The listing builds one solid part. Answer for the finished solid, in the listing's coordinates (mm). A direction names the side the tool comes from. Round coordinates to 2 decimals unless told otherwise and drop trailing zeros. Write each loop counter-clockwise with the first axis right and the second up, starting at its lowest first coordinate (ties: lowest second). Pieces come first, ordered by that corner, then holes.
(1) For faces 4 (the face through (5.07, 345.49, -4.28)), 5 (the face through (25, 312, -25)), 6 (the face through (18, 121, -10)), determine the directions among +Z, -Z, +X, -X, +Y, -Y from which every point of the face is accessible in a straight line to the end or side of a thin tool.
(2) A cutting plane is placed at D-D, the plane x = 4.5. Give the vertices of the cut face in (y, z).
(3) A cutting plane is placed at C-C, the plane y = 325. Give the vertices of the cut face in (x, z), and give its area (3 significant figures).
(4) The mould has two halves that part along Y. Classify faces 1 (the face through (17, 275, -25)), 2 (the face through (17, 0, -25)), 3 (the face through (4.93, 329.957, -25.651)): +Y half, -Y half, draft (parallel to the pull), parting line (faces both ways), or undercut.
(5) This flat-tipped pin is pushed along its axis until it touches: pin 1 Ø7.5 at (x, z) = (20, -23.5) entering from +Y. Where does it stop, or does it pass through?
(6) A cutting plane is placed at A-A, the plane y = 81.5. Give the vertices of the cut face in (x, z).
(7) A cutting plane is placed at B-B, the plane z = -25. Give the vertices of the cut face in (x, y), and give its area (3 significant figures).
(8) Find the intervals of material crossed by probe 1 along Y at (x, z) = (28, -25); probe 2 along Z at (x, y) = (28.75, 325); probe 3 along Z at (x, y) = (9.5, 178), in increasing order.
from build123d import *

# Parameters (mm, degrees)
SKETCH1_W           = 35
SKETCH1_H           = 50
BOSS_EXTRUDE1_DEPTH = 350
CUT_EXTRUDE1_DEPTH  = 350
SKETCH3_W           = 30
SKETCH3_H           = 225
CUT_EXTRUDE2_DEPTH  = 350
SKETCH4_W           = 15
SKETCH4_H           = 75
CUT_EXTRUDE3_DEPTH  = 350
SKETCH5_R           = 5
CUT_EXTRUDE4_DEPTH  = 356.28157847


with BuildPart() as part:
    # Sketch1 → Boss-Extrude1 (new body)
    with BuildSketch(Plane(origin=(0, 0, 0), x_dir=(1, 0, 0), z_dir=(0, 1, 0))):
        with Locations((17.5, 25)):
            Rectangle(SKETCH1_W, SKETCH1_H)
    extrude(amount=BOSS_EXTRUDE1_DEPTH)

    # Sketch2 → Cut-Extrude1 (cut)
    with BuildSketch(Plane(origin=(35, 0, 0), x_dir=(0, 0, -1), z_dir=(1, 0, 0))):
        with BuildLine():
            ThreePointArc((0, 335), (4.393398282, 345.606601718), (15, 350))
            Line((15, 350), (0, 350))
            Line((0, 350), (0, 335))
        make_face()
        with BuildLine():
            Line((50, 350), (35, 350))
            ThreePointArc((35, 350), (45.606601718, 345.606601718), (50, 335))
            Line((50, 335), (50, 350))
        make_face()
    extrude(amount=-CUT_EXTRUDE1_DEPTH, mode=Mode.SUBTRACT)

    # Sketch3 → Cut-Extrude2 (cut)
    with BuildSketch(Plane(origin=(35, 0, 0), x_dir=(0, 0, -1), z_dir=(1, 0, 0))):
        with Locations((25, 122.5)):
            Rectangle(SKETCH3_W, SKETCH3_H)
    extrude(amount=-CUT_EXTRUDE2_DEPTH, mode=Mode.SUBTRACT)

    # Sketch4 → Cut-Extrude3 (cut)
    with BuildSketch(Plane.XY):
        with Locations((17.5, 312.5)):
            Rectangle(SKETCH4_W, SKETCH4_H)
    extrude(amount=-CUT_EXTRUDE3_DEPTH, mode=Mode.SUBTRACT)

    # Sketch5 → Cut-Extrude4 (cut, through all)
    with BuildSketch(Plane.ZY):
        with Locations((-25, 325)):
            Circle(SKETCH5_R)
    extrude(amount=-CUT_EXTRUDE4_DEPTH, mode=Mode.SUBTRACT)


solid = part.part
Solutions:
1. face 4: +Z, +X, -X, +Y
1. face 5: +Z, -Z, +Y
1. face 6: +X, -X
2. outline: (0, -50) - (335, -50) arc R15 ccw to (350, -35) - (350, -15) arc R15 ccw to (335, 0) - (0, 0) - close; hole (10, -40) - (235, -40) - (235, -10) - (10, -10) - close; hole circle Ø10 at (325, -25)
3. outline: (0, -50) - (10, -50) - (10, -30) - (0, -30) - close; (0, -20) - (10, -20) - (10, 0) - (0, 0) - close; (25, -50) - (35, -50) - (35, -30) - (25, -30) - close; (25, -20) - (35, -20) - (35, 0) - (25, 0) - close
3. area: 800 mm2
4. face 1: +Y half
4. face 2: -Y half
4. face 3: undercut
5. pin 1: stops at y = 275
6. outline: (0, -50) - (35, -50) - (35, -40) - (0, -40) - close; (0, -10) - (35, -10) - (35, 0) - (0, 0) - close
7. outline: (0, 0) - (35, 0) - (35, 10) - (0, 10) - close; (0, 235) - (35, 235) - (35, 320) - (25, 320) - (25, 275) - (10, 275) - (10, 320) - (0, 320) - close; (0, 330) - (10, 330) - (10, 350) - (0, 350) - close; (25, 330) - (35, 330) - (35, 350) - (25, 350) - close
7. area: 3,050 mm2
8. probe 1: y = 0 to 10, 235 to 320, 330 to 350
8. probe 2: z = -50 to -30, -20 to 0
8. probe 3: z = -50 to -40, -10 to 0
